```python
from build123d import *

# Parameters (mm, degrees)
BOSS_EXTRUDE2_DEPTH = 1.5875
SKETCH2_R           = 3.2639
CUT_EXTRUDE1_DEPTH  = 795.974704399
FILLET1_R           = 6.35
LPATTERN1_START     = -1.5875
LPATTERN1_OUTLINE_R = 3.2639
LPATTERN1_DEPTH     = 3.175
LPATTERN2_START     = -1.5875
LPATTERN2_OUTLINE_R = 3.2639
LPATTERN2_DEPTH     = 3.175
SKETCH3_R           = 3.2639
CUT_EXTRUDE2_DEPTH  = 795.974704399


# Read off the part's stored shape, not the designer's step: LPattern1, LPattern2
with BuildPart() as part:
    # Sketch1 → Boss-Extrude2 (new, symmetric)
    with BuildSketch(Plane(origin=(0, 0, 0), x_dir=(1, 0, 0), z_dir=(0, 1, 0))):
        Polygon((0, 203.2), (63.5, 203.2), (133.096984938, 133.603015062), (203.2, 63.5), (203.2, 0), (355.203125, 0), (355.203125, 711.2), (203.2, 711.2), (203.2, 647.7), (63.5, 508), (0, 508), align=None)
    extrude(amount=BOSS_EXTRUDE2_DEPTH, both=True)

    # Sketch2 → Cut-Extrude1 (cut, through all)
    with BuildSketch(Plane(origin=(0, 1.5875, 0), x_dir=(1, 0, 0), z_dir=(0, 1, 0))):
        with Locations(Location((209.55, 698.5, 0), (0, 0, 270))):
            Circle(SKETCH2_R)
        with Locations(Location((12.7, 501.65, 0), (0, 0, 270))):
            Circle(SKETCH2_R)
        with Locations(Location((209.55, 12.7, 0), (0, 0, 270))):
            Circle(SKETCH2_R)
    extrude(amount=-CUT_EXTRUDE1_DEPTH, mode=Mode.SUBTRACT)

    # Fillet1
    fillet1_edges = [part.edges().sort_by_distance(p)[0] for p in [
        (0, 0, -508),
        (63.5, 0, -508),
        (203.2, 0, -647.7),
        (203.2, 0, -711.2),
        (355.203125, 0, -711.2),
        (355.203125, 0, 0),
        (203.2, 0, 0),
        (203.2, 0, -63.5),
        (63.5, 0, -203.2),
        (0, 0, -203.2),
    ]]
    fillet(fillet1_edges, radius=FILLET1_R)

    # LPattern1 outline → LPattern1 (cut)
    with BuildSketch(Plane(origin=(0, 0, 0), x_dir=(1, 0, 0), z_dir=(0, 1, 0)).offset(LPATTERN1_START)):
        with Locations((12.7, 209.55)):
            Circle(LPATTERN1_OUTLINE_R)
        with Locations((12.7, 222.25)):
            Circle(LPATTERN1_OUTLINE_R)
        with Locations((12.7, 234.95)):
            Circle(LPATTERN1_OUTLINE_R)
        with Locations((12.7, 247.65)):
            Circle(LPATTERN1_OUTLINE_R)
        with Locations((12.7, 260.35)):
            Circle(LPATTERN1_OUTLINE_R)
        with Locations((12.7, 273.05)):
            Circle(LPATTERN1_OUTLINE_R)
        with Locations((12.7, 285.75)):
            Circle(LPATTERN1_OUTLINE_R)
        with Locations((12.7, 298.45)):
            Circle(LPATTERN1_OUTLINE_R)
        with Locations((12.7, 311.15)):
            Circle(LPATTERN1_OUTLINE_R)
        with Locations((12.7, 323.85)):
            Circle(LPATTERN1_OUTLINE_R)
        with Locations((12.7, 336.55)):
            Circle(LPATTERN1_OUTLINE_R)
        with Locations((12.7, 349.25)):
            Circle(LPATTERN1_OUTLINE_R)
        with Locations((12.7, 361.95)):
            Circle(LPATTERN1_OUTLINE_R)
        with Locations((12.7, 374.65)):
            Circle(LPATTERN1_OUTLINE_R)
        with Locations((12.7, 387.35)):
            Circle(LPATTERN1_OUTLINE_R)
        with Locations((12.7, 400.05)):
            Circle(LPATTERN1_OUTLINE_R)
        with Locations((12.7, 412.75)):
            Circle(LPATTERN1_OUTLINE_R)
        with Locations((12.7, 425.45)):
            Circle(LPATTERN1_OUTLINE_R)
        with Locations((12.7, 438.15)):
            Circle(LPATTERN1_OUTLINE_R)
        with Locations((12.7, 450.85)):
            Circle(LPATTERN1_OUTLINE_R)
        with Locations((12.7, 463.55)):
            Circle(LPATTERN1_OUTLINE_R)
        with Locations((12.7, 476.25)):
            Circle(LPATTERN1_OUTLINE_R)
        with Locations((12.7, 488.95)):
            Circle(LPATTERN1_OUTLINE_R)
    extrude(amount=LPATTERN1_DEPTH, mode=Mode.SUBTRACT)

    # LPattern2 outline → LPattern2 (cut)
    with BuildSketch(Plane(origin=(0, 0, 0), x_dir=(1, 0, 0), z_dir=(0, 1, 0)).offset(LPATTERN2_START)):
        with Locations((349.25, 12.7)):
            Circle(LPATTERN2_OUTLINE_R)
        with Locations((349.25, 698.5)):
            Circle(LPATTERN2_OUTLINE_R)
        with Locations((336.55, 12.7)):
            Circle(LPATTERN2_OUTLINE_R)
        with Locations((336.55, 698.5)):
            Circle(LPATTERN2_OUTLINE_R)
        with Locations((323.85, 12.7)):
            Circle(LPATTERN2_OUTLINE_R)
        with Locations((323.85, 698.5)):
            Circle(LPATTERN2_OUTLINE_R)
        with Locations((311.15, 12.7)):
            Circle(LPATTERN2_OUTLINE_R)
        with Locations((311.15, 698.5)):
            Circle(LPATTERN2_OUTLINE_R)
        with Locations((298.45, 12.7)):
            Circle(LPATTERN2_OUTLINE_R)
        with Locations((298.45, 698.5)):
            Circle(LPATTERN2_OUTLINE_R)
        with Locations((285.75, 12.7)):
            Circle(LPATTERN2_OUTLINE_R)
        with Locations((285.75, 698.5)):
            Circle(LPATTERN2_OUTLINE_R)
        with Locations((273.05, 12.7)):
            Circle(LPATTERN2_OUTLINE_R)
        with Locations((273.05, 698.5)):
            Circle(LPATTERN2_OUTLINE_R)
        with Locations((260.35, 12.7)):
            Circle(LPATTERN2_OUTLINE_R)
        with Locations((260.35, 698.5)):
            Circle(LPATTERN2_OUTLINE_R)
        with Locations((247.65, 12.7)):
            Circle(LPATTERN2_OUTLINE_R)
        with Locations((247.65, 698.5)):
            Circle(LPATTERN2_OUTLINE_R)
        with Locations((234.95, 12.7)):
            Circle(LPATTERN2_OUTLINE_R)
        with Locations((234.95, 698.5)):
            Circle(LPATTERN2_OUTLINE_R)
        with Locations((222.25, 12.7)):
            Circle(LPATTERN2_OUTLINE_R)
        with Locations((222.25, 698.5)):
            Circle(LPATTERN2_OUTLINE_R)
    extrude(amount=LPATTERN2_DEPTH, mode=Mode.SUBTRACT)

    # Sketch3 → Cut-Extrude2 (cut, through all)
    with BuildSketch(Plane(origin=(0, 1.5875, 0), x_dir=(1, 0, 0), z_dir=(0, 1, 0))):
        with Locations(Location((247.65, 698.5, 0), (0, 0, 270))):
            Circle(SKETCH3_R)
        with Locations(Location((247.65, 673.1, 0), (0, 0, 270))):
            Circle(SKETCH3_R)
        with Locations(Location((247.65, 647.7, 0), (0, 0, 270))):
            Circle(SKETCH3_R)
        with Locations(Location((247.65, 622.3, 0), (0, 0, 270))):
            Circle(SKETCH3_R)
        with Locations(Location((247.65, 596.9, 0), (0, 0, 270))):
            Circle(SKETCH3_R)
        with Locations(Location((247.65, 571.5, 0), (0, 0, 270))):
            Circle(SKETCH3_R)
        with Locations(Location((247.65, 546.1, 0), (0, 0, 270))):
            Circle(SKETCH3_R)
        with Locations(Location((247.65, 520.7, 0), (0, 0, 270))):
            Circle(SKETCH3_R)
        with Locations(Location((247.65, 495.3, 0), (0, 0, 270))):
            Circle(SKETCH3_R)
        with Locations(Location((247.65, 469.9, 0), (0, 0, 270))):
            Circle(SKETCH3_R)
        with Locations(Location((247.65, 444.5, 0), (0, 0, 270))):
            Circle(SKETCH3_R)
        with Locations(Location((247.65, 419.1, 0), (0, 0, 270))):
            Circle(SKETCH3_R)
        with Locations(Location((247.65, 393.7, 0), (0, 0, 270))):
            Circle(SKETCH3_R)
        with Locations(Location((247.65, 368.3, 0), (0, 0, 270))):
            Circle(SKETCH3_R)
        with Locations(Location((247.65, 342.9, 0), (0, 0, 270))):
            Circle(SKETCH3_R)
        with Locations(Location((247.65, 317.5, 0), (0, 0, 270))):
            Circle(SKETCH3_R)
        with Locations(Location((247.65, 292.1, 0), (0, 0, 270))):
            Circle(SKETCH3_R)
        with Locations(Location((247.65, 266.7, 0), (0, 0, 270))):
            Circle(SKETCH3_R)
        with Locations(Location((247.65, 241.3, 0), (0, 0, 270))):
            Circle(SKETCH3_R)
        with Locations(Location((247.65, 215.9, 0), (0, 0, 270))):
            Circle(SKETCH3_R)
        with Locations(Location((247.65, 190.5, 0), (0, 0, 270))):
            Circle(SKETCH3_R)
        with Locations(Location((247.65, 165.1, 0), (0, 0, 270))):
            Circle(SKETCH3_R)
        with Locations(Location((247.65, 139.7, 0), (0, 0, 270))):
            Circle(SKETCH3_R)
        with Locations(Location((247.65, 114.3, 0), (0, 0, 270))):
            Circle(SKETCH3_R)
        with Locations(Location((247.65, 88.9, 0), (0, 0, 270))):
            Circle(SKETCH3_R)
        with Locations(Location((247.65, 63.5, 0), (0, 0, 270))):
            Circle(SKETCH3_R)
        with Locations(Location((247.65, 38.1, 0), (0, 0, 270))):
            Circle(SKETCH3_R)
    extrude(amount=-CUT_EXTRUDE2_DEPTH, mode=Mode.SUBTRACT)


solid = part.part
```
The listing builds one solid part. Answer for the finished solid, in the listing's coordinates (mm). Coordinates: 2 decimals unless noted, no trailing zeros. Loops run counter-clockwise (first coordinate to the right, second up) from the corner with the lowest first, then second, coordinate; pieces in that order, holes last. Notation, with made-up numbers: (4.5, 26.25) -> (34.5, 26.25) arc R22 ccw to (34.5, 53.25) -> close; hole circle Ø2 at (87, 66.5). An arc over 180 degrees is marked (long way). Return JSON: item names as keys, results as strings. Group by question number.
(1) A cutting plane is placed at A-A on y = 0.8. Count the separate pieces of the cut face and the enclosed holes in it, and give its area (3 significant figures).
(2) Given pin 1 Ø1 at (y, z) = (0.5, -33.5) entering from -X, flat-ended and moving along its own axis, determine where the tip first touches the part or whether it passes through.
(3) A cutting plane is placed at B-B on x = 142. Write down the section's boundary in (y, z).
(4) A cutting plane is placed at C-C on x = 188. Write down the section's boundary in (y, z), and give its area (3 significant figures).
(5) Find the intervals of material crossed by probe 1 along Z at (x, y) = (272.5, -0.65); probe 2 along Z at (x, y) = (273.05, 0.6); probe 3 along X at (y, z) = (-0.55, -450.85), in increasing order. Write a range as from..to.
The answers:
{
 "1": {"separate pieces": "1", "enclosed holes": "74", "area": "187,000 mm^2"},
 "2": {"pin 1": "stops at x = 203.2"},
 "3": {"outline": "(-1.59, -586.5) -> (1.59, -586.5) -> (1.59, -124.7) -> (-1.59, -124.7) -> close"},
 "4": {"outline": "(-1.59, -632.5) -> (1.59, -632.5) -> (1.59, -78.7) -> (-1.59, -78.7) -> close", "area": "1,760 mm^2"},
 "5": {"probe 1": "z = -711.2..-701.72, -695.28..-15.92, -9.48..0", "probe 2": "z = -711.2..-701.76, -695.24..-15.96, -9.44..0", "probe 3": "x = 0..9.44, 15.96..355.2"}
}
